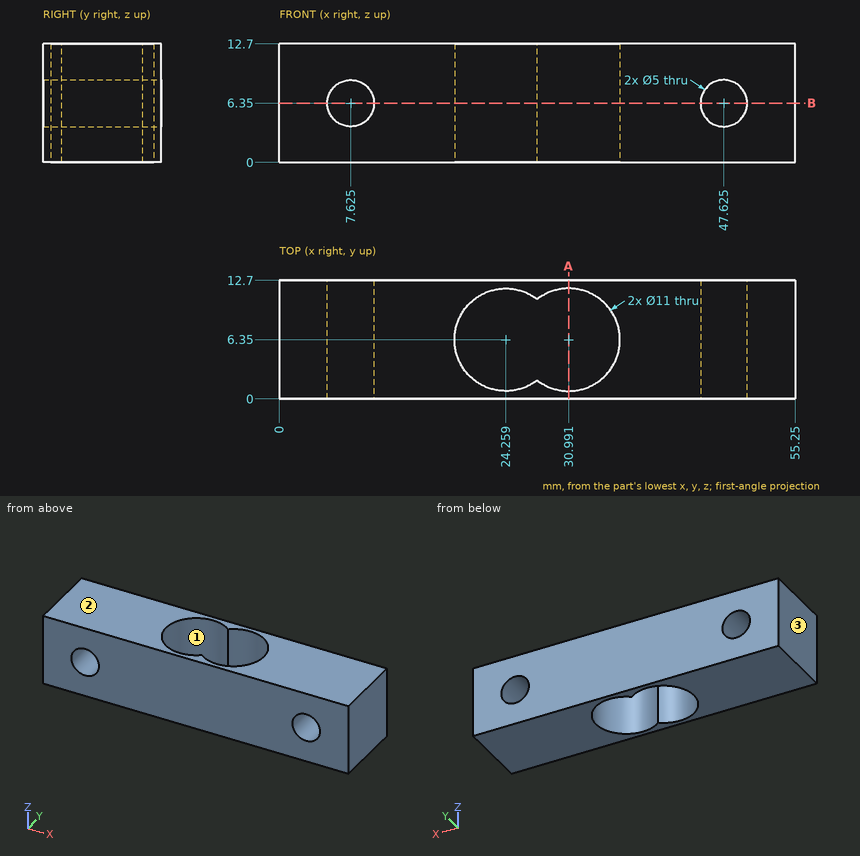
Part print with two shaded views. Sizes in mm from the minimum x, y, z corner. Coordinates: 2 decimals unless noted, no trailing zeros. Write each loop counter-clockwise with the first axis right and the second up, starting at its lowest first coordinate (ties: lowest second). Pieces come first, ordered by that corner, then holes.
1. Drill centre lines: probe 1 along X at (y, z) = (6.35, 6); probe 2 along X at (y, z) = (6, 8.5); probe 3 along X at (y, z) = (3, 1.5). Where is each one in solid material? Low to high.
Answer block:
probe 1: x = 0 to 5.15, 10.1 to 18.76, 36.49 to 45.15, 50.1 to 55.25
probe 2: x = 0 to 6.35, 8.9 to 18.77, 36.48 to 46.35, 48.9 to 55.25
probe 3: x = 0 to 19.9, 35.35 to 55.25
2. Pull direction X, two halves, no side cores. Call the marked faces 1, 2 and 3: released by +X, released by -X, zero draft, split by the parting line, or undercut.
Answer block:
face 1: undercut
face 2: zero draft
face 3: released by -X
3. Band-saw the part on B-B, the plane z = 6.35. Give the number of separate pieces and of enclosed holes in the cut face.
Answer block:
separate pieces: 3
enclosed holes: 1
4. Band-saw the part on A-A, the plane x = 31. Give the cut face in (y, z), and give its area (3 significant figures).
Answer block:
outline: (0, 0) - (0.85, 0) - (0.85, 12.7) - (0, 12.7) - close; (11.85, 0) - (12.7, 0) - (12.7, 12.7) - (11.85, 12.7) - close
area: 21.6 mm2
5. Drop a flat-ended pin along its axis: pin 1 (6 mm diameter, centred on x = 47.625, z = 6.35, fed in from -Y). Give the stop position or say it passes through.
Answer block:
pin 1: stops at y = 0
